Check sheet for the modelled part. Datum: model origin and axes. Units: mm. A direction names the side the tool comes from. Coordinates: 2 decimals unless noted, no trailing zeros. Write each loop counter-clockwise with the first axis right and the second up, starting at its lowest first coordinate (ties: lowest second). Pieces come first, ordered by that corner, then holes. Notation, with made-up numbers: (30.25, 24.25) -> (53.25, 24.25) arc R22 cw to (53.25, 32.25) -> close; hole circle Ø8 at (59, 86). An arc over 180 degrees is marked (long way). Put each result on its own line as item: value.
```python
from build123d import *

# Parameters (mm, degrees)
F0_W            = 59
F0_H            = 59
F3_DEPTH        = 15
F1_W            = 53
F1_H            = 53
F4_DEPTH        = 12
F2_W            = 22
F2_H            = 14
F5_DEPTH        = 30
F5_DEPTH_BACK   = 30
F6_R            = 2
F8_R            = 5
F9_DEPTH        = 6
F11_D           = 4.4
F11_CBORE_D     = 8.25
F11_CBORE_DEPTH = 4
F12_D           = 4.4
F12_CBORE_D     = 8.25
F12_CBORE_DEPTH = 4
F13_D           = 4.4
F13_CBORE_D     = 8.25
F13_CBORE_DEPTH = 4
F14_D           = 4.4
F14_CBORE_D     = 8.25
F14_CBORE_DEPTH = 4


with BuildPart() as f3:
    # F0 (on Front) → F3 (new body)
    with BuildSketch(Plane.XZ):
        Rectangle(F0_W, F0_H)
    extrude(amount=F3_DEPTH)

    # F1 (on Front) → F4 (cut)
    with BuildSketch(Plane.XZ):
        Rectangle(F1_W, F1_H)
    extrude(amount=F4_DEPTH, mode=Mode.SUBTRACT)

    # F2 (on Top) → F5 (cut, two sides)
    with BuildSketch(Plane.XY) as f5_sk:
        Rectangle(F2_W, F2_H)
    extrude(amount=-F5_DEPTH, mode=Mode.SUBTRACT)
    extrude(f5_sk.sketch, amount=F5_DEPTH_BACK, mode=Mode.SUBTRACT)

    # F6
    f6_edges = [f3.edges().sort_by_distance(p)[0] for p in [
        (0, -15, 29.5),
        (-29.5, -15, 0),
        (0, -15, -29.5),
        (29.5, -15, 0),
    ]]
    fillet(f6_edges, radius=F6_R)

    # F8 (on offset) → F9 (join)
    with BuildSketch(Plane.XZ.offset(15)):
        with Locations((19.5, 19.5)):
            Circle(F8_R)
        with Locations((-19.5, 19.5)):
            Circle(F8_R)
        with Locations((19.5, -19.5)):
            Circle(F8_R)
        with Locations((-19.5, -19.5)):
            Circle(F8_R)
    extrude(amount=-F9_DEPTH)

    # F11 (through all)
    with Locations(Plane.XZ.offset(15)):
        with Locations((-19.5, 19.5)):
            CounterBoreHole(F11_D / 2, F11_CBORE_D / 2, F11_CBORE_DEPTH)

    # F12 (through all)
    with Locations(Plane.XZ.offset(15)):
        with Locations((-19.5, -19.5)):
            CounterBoreHole(F12_D / 2, F12_CBORE_D / 2, F12_CBORE_DEPTH)

    # F13 (through all)
    with Locations(Plane.XZ.offset(15)):
        with Locations((19.5, -19.5)):
            CounterBoreHole(F13_D / 2, F13_CBORE_D / 2, F13_CBORE_DEPTH)

    # F14 (through all)
    with Locations(Plane.XZ.offset(15)):
        with Locations((19.5, 19.5)):
            CounterBoreHole(F14_D / 2, F14_CBORE_D / 2, F14_CBORE_DEPTH)


solid = f3.part
```
Q1. Cross-section at B-B (y = -1). Record the cut outline in (x, z).
Recorded:
outline: (-29.5, -29.5) -> (-11, -29.5) -> (-11, -26.5) -> (-26.5, -26.5) -> (-26.5, 26.5) -> (-11, 26.5) -> (-11, 29.5) -> (-29.5, 29.5) -> close; (11, -29.5) -> (29.5, -29.5) -> (29.5, 29.5) -> (11, 29.5) -> (11, 26.5) -> (26.5, 26.5) -> (26.5, -26.5) -> (11, -26.5) -> close
Q2. Cross-section at D-D (z = 9.5). Record the cut outline in (x, y), plus the area to 3 significant figures.
Recorded:
outline: (-29.5, -13) arc R2 ccw to (-27.5, -15) -> (27.5, -15) arc R2 ccw to (29.5, -13) -> (29.5, 0) -> (26.5, 0) -> (26.5, -12) -> (-26.5, -12) -> (-26.5, 0) -> (-29.5, 0) -> close
area: 247 mm2
Q3. Mould release check, pull along Z, two halves, no side actions. Record for faces 1 (the cylindrical face through (0.41, -14.4, 28.93)), 2 (the flat face through (11, -4, 28)), 3 (the cylindrical face through (18.42, -10.52, 14.62)), 4 (the flat face through (0, -8, -29.5)): released by +Z, released by -Z, zero draft, split by the parting line, or undercut.
Recorded:
face 1: released by +Z
face 2: zero draft
face 3: undercut
face 4: released by -Z
Q4. Cross-section at A-A (x = 19.5). State how many separate pieces and enclosed holes the cut face has, plus the area to 3 significant figures.
Recorded:
separate pieces: 3
enclosed holes: 0
area: 224 mm2
Q5. Material ranges on line 1 along Z through (x, y) = (19.5, -9.5); line 2 along Z through (x, y) = (19.5, -13.1) (1 decimal); line 3 along Z through (x, y) = (16.5, -2), recorded low to high.
Recorded:
line 1: z = -29.5 to -26.5, -24.5 to -21.7, -17.3 to -14.5, 14.5 to 17.3, 21.7 to 24.5, 26.5 to 29.5
line 2: z = -29.5 to -23.6, -15.4 to 15.4, 23.6 to 29.5
line 3: z = -29.5 to -26.5, 26.5 to 29.5
Q6. Tool access check on faces 5 (the cylindrical face through (16.46, -13.03, -16.71)), 6 (the cylindrical face through (-20.58, -10.52, 14.62)), 7 (the flat face through (-11, -4, 28)). Record the directions out of +Z, -Z, +X, -X, +Y, -Y that give a thin tool (end or side, any length) a straight path to the whole face; none if there is none.
Recorded:
face 5: -Y
face 6: +Y
face 7: +Z, -Z, +Y
Q7. Depth check by flat-ended pin: P1, Ø4, axis at x = 19.5, z = 20, coming from the -Y side; P2, Ø3, axis at x = -18, z = -19, coming from the +Y side; P3, Ø1.5, axis at x = -1.5, z = 27.5, coming from the +Y side. Enter the tip coordinate at first touch or a pass-through.
Recorded:
P1: stops at y = -11
P2: stops at y = -9
P3: stops at y = -7
